For this review, take the finished solid that the model builds, in its own axes (mm). A direction names the side the tool comes from. Give positions to 0.01 mm unless a question says otherwise; leave off trailing zeros. Write each loop counter-clockwise with the first axis right and the second up, starting at its lowest first coordinate (ties: lowest second). Pieces come first, ordered by that corner, then holes. Notation, with made-up numbers: (77.25, 79) -> (102.25, 79) arc R19 cw to (102.25, 98) -> close; hole circle Ø3 at (8.5, 84.5). An arc over 180 degrees is marked (long way). Write item = value, one per line.
```python
from build123d import *

# Parameters (mm, degrees)
F0_W     = 152.4
F0_H     = 152.4
F1_DEPTH = 2286
F2_W     = 25.4
F2_H     = 914.4
F2_H_2   = 304.8
F3_DEPTH = 533.4
F5_W     = 1219.2
F5_H     = 152.4
F5_W_2   = 152.4
F6_DEPTH = 38.1


with BuildPart() as f1:
    # F0 (on Top) → F1 (new body)
    with BuildSketch(Plane.XY):
        with Locations((76.2, -76.2)):
            Rectangle(F0_W, F0_H)
    extrude(amount=F1_DEPTH)

    # F2 (on face) → F3 (join)
    with BuildSketch(Plane.YZ.offset(152.4)):
        with Locations((-76.2, 1219.2)):
            Rectangle(F2_W, F2_H)
        with Locations((-76.2, 1981.2)):
            Rectangle(F2_W, F2_H_2)
    extrude(amount=F3_DEPTH)

    # F4: F1 across face


with BuildPart() as f1_1:
    add(f1.part)
    add(f1.part.mirror(Plane(origin=(685.8, -76.2, 1219.2), x_dir=(0, 1, 0), z_dir=(1, 0, 0))))

    # F5 (on face) → F6 (join)
    with BuildSketch(Plane.XZ.offset(152.4)):
        with Locations((762, 2209.8)):
            Rectangle(F5_W, F5_H)
        with Locations((76.2, 2209.8)):
            Rectangle(F5_W_2, F5_H)
    extrude(amount=F6_DEPTH)


solid = f1_1.part
```
(1) Tool access review of faces 1 (the face through (75, -75, 0)), 2 (the face through (1296, -152.4, 1052)), 3 (the face through (693, -88.9, 1213)), 4 (the face through (693, -63.5, 1213)), 5 (the face through (75, 0, 1127)): name each direction out of +Z, -Z, +X, -X, +Y, -Y from which nothing blocks a thin tool from reaching the whole face with its end or side.
Answers below:
face_1 = -Z, +X, -X, +Y, -Y
face_2 = -Z, +X, -X, -Y
face_3 = +Z, -Z, -Y
face_4 = +Z, -Z, +Y
face_5 = +Z, -Z, +X, -X, +Y
(2) Take a section at A-A (y = -36). Write out the cut boundary in (x, z), plus the area to 3 significant figures.
Answers below:
outline = (0, 0) -> (152.4, 0) -> (152.4, 2286) -> (0, 2286) -> close; (1219.2, 0) -> (1371.6, 0) -> (1371.6, 2286) -> (1219.2, 2286) -> close
area = 697,000 mm^2
(3) To check wall thickness, follow probe 1 along X at (y, z) = (-138, 1338); probe 2 along Z at (x, y) = (219.5, -73.5); probe 3 along Y at (x, z) = (503.5, 1430.5). State the ranges of each line that lie inside material, in increasing order.
Answers below:
probe_1 = 0 to 152.4, 1219.2 to 1371.6
probe_2 = 762 to 1676.4, 1828.8 to 2133.6
probe_3 = -88.9 to -63.5
(4) Take a section at B-B (x = 1163). Write out the cut boundary in (y, z).
Answers below:
outline = (-190.5, 2133.6) -> (-152.4, 2133.6) -> (-152.4, 2286) -> (-190.5, 2286) -> close; (-88.9, 762) -> (-63.5, 762) -> (-63.5, 1676.4) -> (-88.9, 1676.4) -> close; (-88.9, 1828.8) -> (-63.5, 1828.8) -> (-63.5, 2133.6) -> (-88.9, 2133.6) -> close
(5) For pin 1 (12.5 mm diameter, centred on x = 805.5, y = -74, fed in from +Z); pin 2 (6 mm diameter, centred on x = 467.5, y = -149.5, fed in from -Z); pin 3 (5 mm diameter, centred on x = 664.5, z = 1413.5, fed in from -Y), all flat-tipped, find the tip position at first contact; note any pin that passes through.
Answers below:
pin_1 = 2133.6
pin_2 = 2133.6
pin_3 = -88.9
(6) Take a section at C-C (z = 1129). Write out the cut boundary in (x, y), plus the area to 3 significant figures.
Answers below:
outline = (0, -152.4) -> (152.4, -152.4) -> (152.4, -88.9) -> (1219.2, -88.9) -> (1219.2, -152.4) -> (1371.6, -152.4) -> (1371.6, 0) -> (1219.2, 0) -> (1219.2, -63.5) -> (152.4, -63.5) -> (152.4, 0) -> (0, 0) -> close
area = 73,500 mm^2
